Part model, mm, in its own coordinate system. Face numbers are marked on the shaded views. A direction names the side the tool comes from. Round coordinates to 2 decimals unless told otherwise and drop trailing zeros. Order: outer loops, then holes, each group sorted by start corner. A loop starts at its lowest first (then second) coordinate and runs counter-clockwise, first axis right, second up. Notation, with made-up numbers: (25.25, 53.25) - (71.25, 53.25) arc R31 cw to (71.25, 77.25) - close; hole circle Ø7 at (74.25, 34.5). An arc over 180 degrees is marked (long way). Return JSON: item names as keys, results as strings. Group by question number.
Item 1: Drop flat-ended pins along their axis: pin 1 (6 mm diameter, centred on x = 15, z = 19, fed in from -Y); pin 2 (8 mm diameter, centred on x = 29.5, y = -71.5, fed in from +Z). Give the stop position or say it passes through.
Item 2: Saw through at C-C on y = 0. List the corners of the cut face in (x, z), and give its area (3 significant figures).
Item 3: Probe probe 1 along Z at (x, y) = (-17, 19); probe 2 along Z at (x, y) = (33.5, 52); probe 3 along Y at (x, z) = (1, 111). List the from-to ranges inside material, lowest first.
Item 4: Two-plate mould, pull along Z, no slides. Class the marked faces 4, 5 and 6: released by +Z, released by -Z, zero draft, split by the parting line, or undercut.
Item 5: Saw through at A-A on x = -23. List the corners of the cut face in (y, z), and give its area (3 significant figures).
Item 6: Saw through at D-D on x = 7. List the corners of the cut face in (y, z), and give its area (3 significant figures).
Item 7: Saw through at B-B on z = 142. List the corners of the cut face in (x, y).
Item 8: Tool access for the marked faces 1, 2 and 3: list every direction of +Z, -Z, +X, -X, +Y, -Y with a clear straight run to the whole face (end or side of a thin tool).
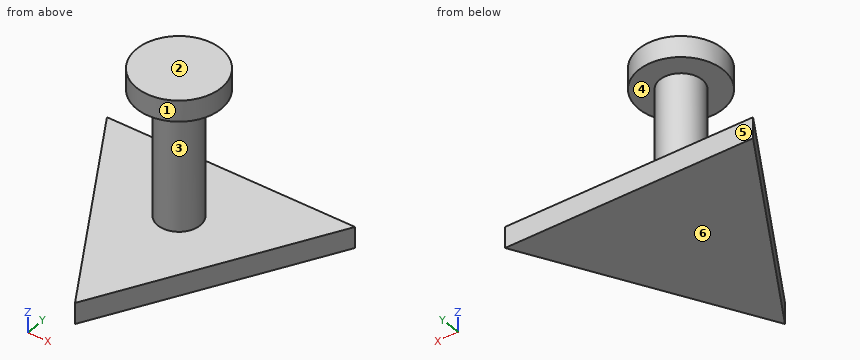
```python
from build123d import *

# Parameters (mm, degrees)
F1_DEPTH = 19.05
F2_R     = 19.05
F3_DEPTH = 114.3
F4_R     = 38.1
F4_R_2   = 19.05
F5_DEPTH = 19.05


with BuildPart() as f1:
    # F0 (on Top) → F1 (new body)
    with BuildSketch(Plane.XY):
        Polygon((-109.985226, 63.5), (0, -127), (109.985226, 63.5), align=None)
    extrude(amount=F1_DEPTH)

    # F2 (on face) → F3 (join)
    with BuildSketch(Plane.XY.offset(19.05)):
        Circle(F2_R)
    extrude(amount=F3_DEPTH)

    # F4 (on face) → F5 (join)
    with BuildSketch(Plane.XY.offset(133.35)):
        Circle(F4_R)
        Circle(F4_R_2, mode=Mode.SUBTRACT)
        Circle(F4_R_2)
    extrude(amount=F5_DEPTH)


solid = f1.part
```
Filled in:
{
 "1": {"pin 1": "stops at y = -106.22", "pin 2": "stops at z = 19.05"},
 "2": {"outline": "(-73.32, 0) - (73.32, 0) - (73.32, 19.05) - (19.05, 19.05) - (19.05, 133.35) - (38.1, 133.35) - (38.1, 152.4) - (-38.1, 152.4) - (-38.1, 133.35) - (-19.05, 133.35) - (-19.05, 19.05) - (-73.32, 19.05) - close", "area": "8,600 mm^2"},
 "3": {"probe 1": "z = 0 to 19.05, 133.35 to 152.4", "probe 2": "z = 0 to 19.05", "probe 3": "y = -19.02 to 19.02"},
 "4": {"face 4": "undercut", "face 5": "zero draft", "face 6": "released by -Z"},
 "5": {"outline": "(-87.16, 0) - (63.5, 0) - (63.5, 19.05) - (-87.16, 19.05) - close; (-30.37, 133.35) - (30.37, 133.35) - (30.37, 152.4) - (-30.37, 152.4) - close", "area": "4,030 mm^2"},
 "6": {"outline": "(-114.88, 0) - (63.5, 0) - (63.5, 19.05) - (17.72, 19.05) - (17.72, 133.35) - (37.45, 133.35) - (37.45, 152.4) - (-37.45, 152.4) - (-37.45, 133.35) - (-17.72, 133.35) - (-17.72, 19.05) - (-114.88, 19.05) - close", "area": "8,880 mm^2"},
 "7": {"outline": "circle Ø76.2 at (0, 0)"},
 "8": {"face 1": "+Z", "face 2": "+Z, +X, -X, +Y, -Y", "face 3": "none"}
}
